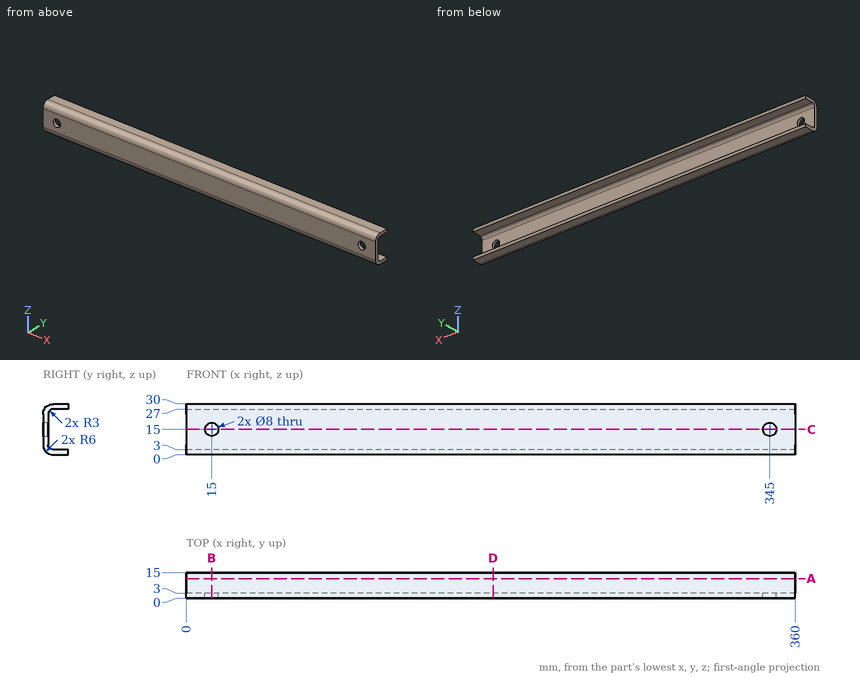
Geometry check sheet. Reference: drawing and pictorial views, mm from the part's lowest x, y, z. Give positions to 0.01 mm unless a question says otherwise; leave off trailing zeros. Loops run counter-clockwise (first coordinate to the right, second up) from the corner with the lowest first, then second, coordinate; pieces in that order, holes last. Notation, with made-up numbers: (46.5, 52) - (94.5, 52) arc R23 cw to (94.5, 63) - close; hole circle Ø4 at (50, 8.5). An arc over 180 degrees is marked (long way). One line per question, with ' | ' between items. Start each with the question number.
1. Gauge pin test, flat ends, axial feed: pin 1 Ø10.5 at (x, z) = (345, 15) entering from +Y; pin 2 Ø8 at (x, z) = (237, 22.5) entering from +Y. Record the tip position at first contact, or that the pin passes through.
2. Cross-section at C-C, the plane z = 15. Enter the section's corners in (x, y), plus the area to 3 significant figures.
3. Cross-section at A-A, the plane y = 11.5. Enter the section's corners in (x, z).
4. Material ranges on line 1 along X through (y, z) = (1.75, 15); line 2 along Z through (x, y) = (266, 13); line 3 along Y through (x, z) = (196, 19.25), recorded low to high. Write a range as [from, to].
5. Cross-section at D-D, the plane x = 181.5. Enter the section's corners in (y, z).
6. Cross-section at B-B, the plane x = 15. Enter the section's corners in (y, z).
Check result:
1) pin 1: stops at y = 3 | pin 2: stops at y = 4.34
2) outline: (0, 0) - (11, 0) - (11, 3) - (0, 3) - close; (19, 0) - (341, 0) - (341, 3) - (19, 3) - close; (349, 0) - (360, 0) - (360, 3) - (349, 3) - close | area: 1,030 mm2
3) outline: (0, 0) - (360, 0) - (360, 3) - (0, 3) - close; (0, 27) - (360, 27) - (360, 30) - (0, 30) - close
4) line 1: x = [0, 11], [19, 341], [349, 360] | line 2: z = [0, 3], [27, 30] | line 3: y = [0, 3]
5) outline: (0, 6) arc R6 ccw to (6, 0) - (15, 0) - (15, 3) - (6, 3) arc R3 cw to (3, 6) - (3, 24) arc R3 cw to (6, 27) - (15, 27) - (15, 30) - (6, 30) arc R6 ccw to (0, 24) - close
6) outline: (0, 6) arc R6 ccw to (6, 0) - (15, 0) - (15, 3) - (6, 3) arc R3 cw to (3, 6) - (3, 11) - (0, 11) - close; (0, 19) - (3, 19) - (3, 24) arc R3 cw to (6, 27) - (15, 27) - (15, 30) - (6, 30) arc R6 ccw to (0, 24) - close
